from build123d import *

# Parameters (mm, degrees)
F2_R     = 6.5
F3_DEPTH = 23
F4_SIZE  = 1
F5_R     = 2


with BuildPart() as f1:
    # F0 (on Front) → F1 (revolve)
    with BuildSketch(Plane.XZ):
        with BuildLine():
            Line((98.207469, 0), (0, 0))
            Line((0, 0), (0, -10))
            Line((0, -10), (13, -10))
            ThreePointArc((13, -10), (24.08707, -8.287742), (35.019375, -10.805614))
            ThreePointArc((35.019375, -10.805614), (65.095188, -16.160515), (94.245718, -7.02399))
            ThreePointArc((94.245718, -7.02399), (97.148746, -4.032118), (98.207469, 0))
        make_face()
    revolve(axis=Axis((-34.182759, 0, 0), (1, 0, 0)))

    # F2 (on face) → F3 (join)
    with BuildSketch(Plane(origin=(0, 0, 0), x_dir=(0, -1, 0), z_dir=(-1, 0, 0))):
        Circle(F2_R)
    extrude(amount=F3_DEPTH)

    # F4
    f4_edges = [f1.edges().sort_by_distance(p)[0] for p in [
        (-23, 6.5, 0),
    ]]
    chamfer(f4_edges, length=F4_SIZE)

    # F5
    f5_edges = [f1.edges().sort_by_distance(p)[0] for p in [
        (0, 0, 10),
    ]]
    fillet(f5_edges, radius=F5_R)


solid = f1.part
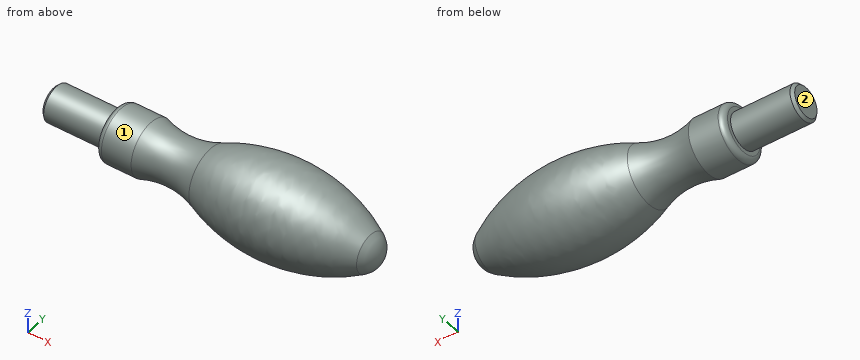
Work out the finished part from the listing and answer in its coordinate system (mm). Face numbers are marked on the shaded views. A direction names the side the tool comes from. Give positions to 0.01 mm unless a question says otherwise; leave off trailing zeros. Loops run counter-clockwise (first coordinate to the right, second up) from the corner with the lowest first, then second, coordinate; pieces in that order, holes last. Notation, with made-up numbers: (39.25, 31) -> (75.25, 31) arc R24 cw to (75.25, 50) -> close; hole circle Ø7 at (-27.5, 0.5). An arc over 180 degrees is marked (long way). Use a Markdown table: item, result. Add a question column.
1) The part is cut by section B-B, the plane x = 20. Determine the outline of the cut face in (y, z).
2) Consider line 1 along Y through (x, z) = (13, -6); line 2 along Y through (x, z) = (77.5, 6); line 3 along Z through (x, y) = (39, 4.5). Determine where each line is inside the solid, lowest interval first.
3) Which of the six approach directions +Z, -Z, +X, -X, +Y, -Y give full straight-line access (tool end or side, diameter ignored) to the marked faces 1 and 2?
4) The part is cut by section A-A, the plane x = 7.5. Determine the outline of the cut face in (y, z), plus the area to 3 significant figures.
5) Each of these flat-tipped pins is pushed along its axis until it touches: P1, Ø6, axis at y = -7.5, z = 1.5, coming from the +X side; P2, Ø3, axis at x = -3.5, z = 1.5, coming from the +Y side; P3, Ø1, axis at x = 3, y = -9, coming from the -Z side; P4, Ø1, axis at x = 2, z = 11.5, coming from the -Y side. Where does it stop, or does it pass through?
Reported:
| question | item | result |
|---|---|---|
| 1 | outline | circle Ø16.84 at (0, 0) |
| 2 | line 1 | y = -8 to 8 |
| 2 | line 2 | y = -12.8 to 12.8 |
| 2 | line 3 | z = -11.56 to 11.56 |
| 3 | face 1 | -X |
| 3 | face 2 | +Z, -Z, -X, +Y, -Y |
| 4 | outline | circle Ø20 at (0, 0) |
| 4 | area | 314 mm^2 |
| 5 | P1 | stops at x = 96.76 |
| 5 | P2 | stops at y = 6.5 |
| 5 | P3 | stops at z = -5.27 |
| 5 | P4 | passes through |
